Input: part model. Units: mm. Frame: model coordinates. Coordinates: 2 decimals unless noted, no trailing zeros. Loops run counter-clockwise (first coordinate to the right, second up) from the corner with the lowest first, then second, coordinate; pieces in that order, holes last. Notation, with made-up numbers: (14, -17) -> (55, -17) arc R23 cw to (55, 8) -> close; hole circle Ø11 at (26, 72). An arc over 180 degrees is marked (long way). Answer as a JSON object with one key per item and string values.
from build123d import *

# Parameters (mm, degrees)
F0_R     = 133.35
F0_R_2   = 38.1
F1_DEPTH = 12.7
F2_R     = 1.27
F4_D     = 10.0838


with BuildPart() as f1:
    # F0 (on Top) → F1 (new body)
    with BuildSketch(Plane.XY):
        Circle(F0_R)
        Circle(F0_R_2, mode=Mode.SUBTRACT)
    extrude(amount=F1_DEPTH)

    # F2
    f2_edges = [f1.edges().sort_by_distance(p)[0] for p in [
        (-38.1, 0, 12.7),
        (-38.1, 0, 0),
        (-133.35, 0, 12.7),
        (-133.35, 0, 0),
    ]]
    fillet(f2_edges, radius=F2_R)

    # F4 (through all)
    with Locations(Plane(origin=(0, 0, 0), x_dir=(1, 0, 0), z_dir=(0, 0, -1))):
        with Locations((0, -120.65), (-104.4859649666, -60.325), (-104.4859649666, 60.325), (0, 120.65), (104.4859649666, 60.325), (104.4859649666, -60.325)):
            Hole(F4_D / 2)


solid = f1.part
1. Pin query (flat end, axial travel): P1, Ø4, axis at x = 51, z = 1.5, coming from the -Y side; P2, Ø4, axis at x = -105.5, z = 6, coming from the -Y side; P3, Ø5, axis at y = 68, z = 8.5, coming from the +X side. Return the tip coordinate at first contact, or that it passes through.
Reply:
{"P1": "stops at y = -124.02", "P2": "stops at y = -84.08", "P3": "stops at x = 116.15"}
2. Section query B-B (x = 0). Return loops of the section in (y, z).
Reply:
{"outline": "(-133.35, 1.27) arc R1.27 ccw to (-132.08, 0) -> (-125.69, 0) -> (-125.69, 12.7) -> (-132.08, 12.7) arc R1.27 ccw to (-133.35, 11.43) -> close; (-115.61, 0) -> (-39.37, 0) arc R1.27 ccw to (-38.1, 1.27) -> (-38.1, 11.43) arc R1.27 ccw to (-39.37, 12.7) -> (-115.61, 12.7) -> close; (38.1, 1.27) arc R1.27 ccw to (39.37, 0) -> (115.61, 0) -> (115.61, 12.7) -> (39.37, 12.7) arc R1.27 ccw to (38.1, 11.43) -> close; (125.69, 0) -> (132.08, 0) arc R1.27 ccw to (133.35, 1.27) -> (133.35, 11.43) arc R1.27 ccw to (132.08, 12.7) -> (125.69, 12.7) -> close"}
3. Section query C-C (z = 3.75). Return loops of the section in (x, y) (3 decimals), plus the area to 3 significant figures.
Reply:
{"outline": "circle Ø266.7 at (0, 0); hole circle Ø10.084 at (-104.486, -60.325); hole circle Ø10.084 at (-104.486, 60.325); hole circle Ø76.2 at (0, 0); hole circle Ø10.084 at (0, -120.65); hole circle Ø10.084 at (0, 120.65); hole circle Ø10.084 at (104.486, -60.325); hole circle Ø10.084 at (104.486, 60.325)", "area": "50,800 mm2"}
4. Section query A-A (y = 0). Return loops of the section in (x, z).
Reply:
{"outline": "(-133.35, 1.27) arc R1.27 ccw to (-132.08, 0) -> (-39.37, 0) arc R1.27 ccw to (-38.1, 1.27) -> (-38.1, 11.43) arc R1.27 ccw to (-39.37, 12.7) -> (-132.08, 12.7) arc R1.27 ccw to (-133.35, 11.43) -> close; (38.1, 1.27) arc R1.27 ccw to (39.37, 0) -> (132.08, 0) arc R1.27 ccw to (133.35, 1.27) -> (133.35, 11.43) arc R1.27 ccw to (132.08, 12.7) -> (39.37, 12.7) arc R1.27 ccw to (38.1, 11.43) -> close"}
5. Line query: line 1 along Y through (x, z) = (0, 4.5); line 2 along X through (y, z) = (24, 9.75); line 3 along Y through (x, z) = (16, 1.5). Output: solid intervals per line, ascending.
Reply:
{"line 1": "y = -133.35 to -125.69, -115.61 to -38.1, 38.1 to 115.61, 125.69 to 133.35", "line 2": "x = -131.17 to -29.59, 29.59 to 131.17", "line 3": "y = -132.39 to -34.58, 34.58 to 132.39"}
6. Mould query, pull axis X, two halves, no side actions, for faces 1 (the face through (127.192, 40.055, 6.279)), 2 (the face through (-31, -28, 12.7)), 3 (the face through (-100.485, 63.393, 6.439)). Classes: pulls with the +X half, pulls with the -X half, needs draft (parallel to the pull), parting line crosses it, or undercut.
Reply:
{"face 1": "parting line crosses it", "face 2": "needs draft", "face 3": "undercut"}
